Can you work these out from the drawing? Everything is in mm from the part's minimum corner. A direction names the side the tool comes from. Give positions to 0.01 mm unless a question says otherwise; leave off trailing zeros. Order: outer loops, then holes, each group sorted by start corner. A loop starts at its lowest first (then second) coordinate and runs counter-clockwise, first axis right, second up. Notation, with made-up numbers: M -37.75,65 L -18.75,65 A31 ccw -18.75,103 Z; hole C 67,-6 d2. An arc over 180 degrees is marked long. Answer as a JSON object with one key per item and string values.
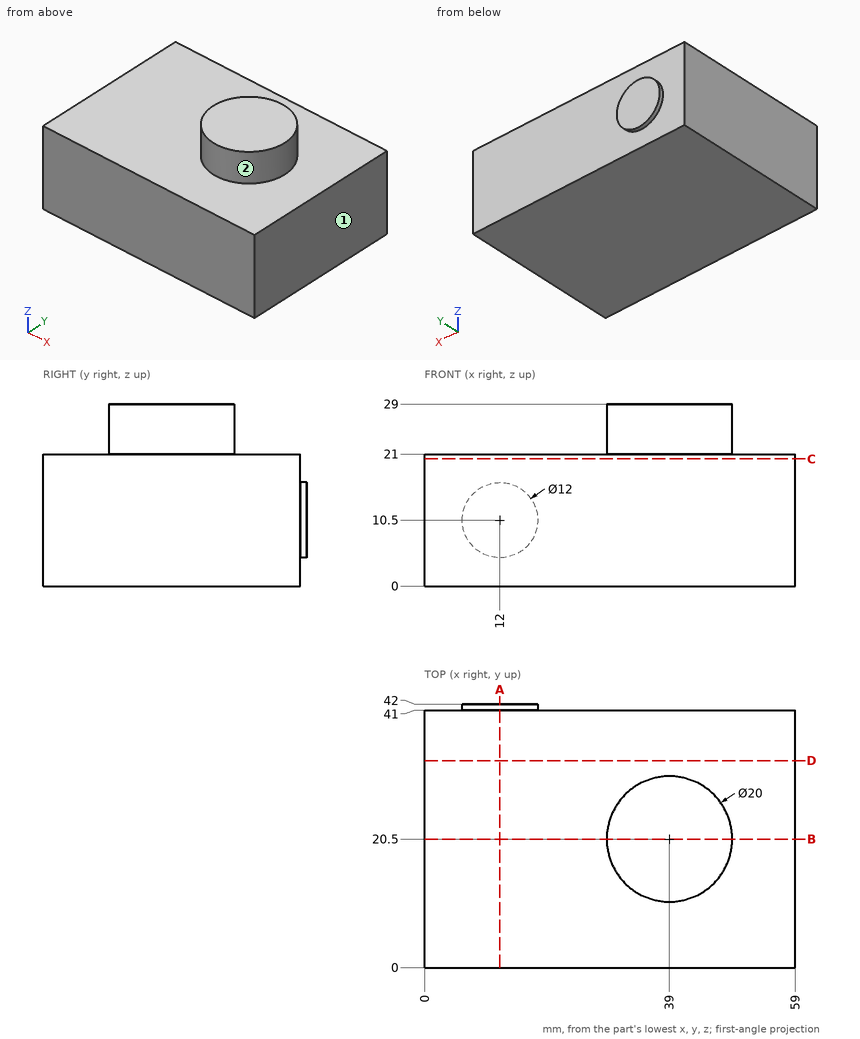
1) For the marked faces 1 and 2, which set-ups out of +Z, -Z, +X, -X, +Y, -Y let a thin tool reach every point of the face, with its end or its side?
Results found:
{"face 1": "+Z, -Z, +X, +Y, -Y", "face 2": "+Z"}
2) I'm going to push flat-ended pins straight in: pin 1 Ø2 at (x, z) = (32.5, 14) entering from -Y; pin 2 Ø1 at (x, y) = (48, 9) entering from +Z; pin 3 Ø2 at (x, z) = (24.5, 3.5) entering from +Y. Where does each tip first touch, or does it pass through?
Results found:
{"pin 1": "stops at y = 0", "pin 2": "stops at z = 21", "pin 3": "stops at y = 41"}
3) I want a section at D-D on y = 33. Write out the boundary of the cut face in (x, z), and give its area (3 significant figures).
Results found:
{"outline": "M 0,0 L 59,0 L 59,21 L 0,21 Z", "area": "1,240 mm²"}
4) I need wall thicknesses on L1, parallel to Y at x = 34, z = 5; L2, parallel to Z at x = 26.5, y = 40.5; L3, parallel to X at y = 23.5, z = 22.5. Which ranges of each line are inside material? Lowest first, please.
Results found:
{"L1": "y = 0 to 41", "L2": "z = 0 to 21", "L3": "x = 29.46 to 48.54"}
5) I want a section at C-C on z = 20.25. Write out the boundary of the cut face in (x, y).
Results found:
{"outline": "M 0,0 L 59,0 L 59,41 L 0,41 Z"}
6) I want a section at B-B on y = 20.5. Write out the boundary of the cut face in (x, z), and give its area (3 significant figures).
Results found:
{"outline": "M 0,0 L 59,0 L 59,21 L 49,21 L 49,29 L 29,29 L 29,21 L 0,21 Z", "area": "1,400 mm²"}
7) I want a section at A-A on x = 12. Write out the boundary of the cut face in (y, z).
Results found:
{"outline": "M 0,0 L 41,0 L 41,4.5 L 42,4.5 L 42,16.5 L 41,16.5 L 41,21 L 0,21 Z"}
